Verification items for the finished model (mm, model axes). Face numbers are marked on the shaded views. A direction names the side the tool comes from. Round coordinates to 2 decimals unless told otherwise and drop trailing zeros. Order: outer loops, then holes, each group sorted by start corner. A loop starts at its lowest first (then second) coordinate and runs counter-clockwise, first axis right, second up. Notation, with made-up numbers: (-28.5, 69.5) -> (-9.5, 69.5) arc R19 cw to (-9.5, 74.5) -> close; hole circle Ø10 at (12.25, 71.5). An arc over 180 degrees is marked (long way). Return JSON: item names as keys, results as strings. Group by question number.
Item 1: Depth check by flat-ended pin: pin 1 Ø1.8 at (x, z) = (-5, -12.5) entering from -Y; pin 2 Ø3 at (x, y) = (6, 12) entering from -Z; pin 3 Ø12 at (x, y) = (2.5, 13.5) entering from +Z; pin 4 Ø2 at (y, z) = (9.5, -6.5) entering from -X. Enter the tip coordinate at first touch or a pass-through.
Item 2: Sectioned sample at A-A on z = 12.5. Record the cut outline in (x, y).
Item 3: Scan lines: probe 1 along Z at (x, y) = (-5.5, 3.5); probe 2 along X at (y, z) = (2.25, -12.5); probe 3 along Z at (x, y) = (-4.75, 14.25). Record each from-to range of solid material in increasing order. Write a range as from..to.
Item 4: Sectioned sample at C-C on y = 18. Record the cut outline in (x, z), plus the area to 3 significant figures.
Item 5: Access from +Z, -Z, +X, -X, +Y, -Y to the whole of each face (thin tool, end or side, straight path). Record for the marked faces 1, 2 and 3.
Item 6: Sectioned sample at B-B on x = -3. Record the cut outline in (y, z).
```python
from build123d import *

# Parameters (mm, degrees)
SKETCH_1_W          = 30
SKETCH_1_H          = 32
EXTRUDE_1_DEPTH     = 6
SKETCH_2_W          = 6
SKETCH_2_H          = 32
EXTRUDE_2_DEPTH     = 20
SKETCH_4_R          = 1.5
CUT_EXTRUDE_1_DEPTH = 30.681644159
SKETCH_5_W          = 24
SKETCH_5_H          = 5
EXTRUDE_3_DEPTH     = 20
CUT_EXTRUDE_2_DEPTH = 36.259750425


with BuildPart() as part:
    # 草图1 → 凸台-拉伸1 (new body)
    with BuildSketch(Plane(origin=(0, 0, 0), x_dir=(1, 0, 0), z_dir=(0, 1, 0))):
        Rectangle(SKETCH_1_W, SKETCH_1_H)
    extrude(amount=EXTRUDE_1_DEPTH)

    # 草图2 → 凸台-拉伸2 (add)
    with BuildSketch(Plane(origin=(0, 6, 0), x_dir=(1, 0, 0), z_dir=(0, 1, 0))):
        with Locations((12, 0)):
            Rectangle(SKETCH_2_W, SKETCH_2_H)
    extrude(amount=EXTRUDE_2_DEPTH)

    # 草图4 → 切除-拉伸1 (cut, through all)
    with BuildSketch(Plane(origin=(0, 6, 0), x_dir=(1, 0, 0), z_dir=(0, 1, 0))):
        with Locations(Location((-5, 12.5, 0), (0, 0, 270))):
            Circle(SKETCH_4_R)
        with Locations(Location((-5, -12.5, 0), (0, 0, 90))):
            Circle(SKETCH_4_R)
    extrude(amount=-CUT_EXTRUDE_1_DEPTH, mode=Mode.SUBTRACT)

    # 草图5 → 凸台-拉伸3 (add, through all)
    with BuildSketch(Plane(origin=(0, 6, 0), x_dir=(1, 0, 0), z_dir=(0, 1, 0))):
        with Locations((-3, 0)):
            Rectangle(SKETCH_5_W, SKETCH_5_H)
    extrude(amount=EXTRUDE_3_DEPTH)

    # 草图6 → 切除-拉伸2 (cut, through all)
    with BuildSketch(Plane.XY.offset(2.5)):
        Polygon((-15, 6), (-15, 26), (9, 26), align=None)
    extrude(amount=-CUT_EXTRUDE_2_DEPTH, mode=Mode.SUBTRACT)


solid = part.part
```
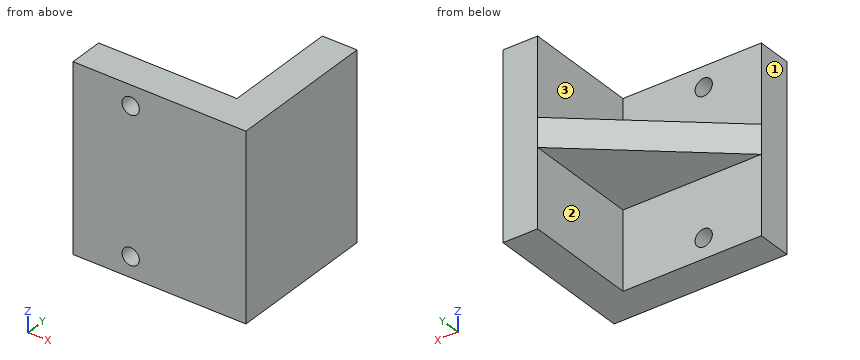
Recorded:
{
 "1": {"pin 1": "through", "pin 2": "z = -2.5", "pin 3": "z = 2.5", "pin 4": "x = 9"},
 "2": {"outline": "(-15, 0) -> (-6.5, 0) -> (-6.5, 6) -> (-15, 6) -> close; (-3.5, 0) -> (15, 0) -> (15, 26) -> (9, 26) -> (9, 6) -> (-3.5, 6) -> close"},
 "3": {"probe 1": "-16..-13.91, -11.09..11.09, 13.91..16", "probe 2": "-15..-6.5, -3.5..15", "probe 3": "-2.5..2.5"},
 "4": {"outline": "(-0.6, -2.5) -> (9, -2.5) -> (9, -16) -> (15, -16) -> (15, 16) -> (9, 16) -> (9, 2.5) -> (-0.6, 2.5) -> close", "area": "240 mm²"},
 "5": {"face 1": "+Z, -Z, -X, +Y, -Y", "face 2": "-Z, -X, +Y", "face 3": "+Z, -X, +Y"},
 "6": {"outline": "(0, -16) -> (6, -16) -> (6, -2.5) -> (16, -2.5) -> (16, 2.5) -> (6, 2.5) -> (6, 16) -> (0, 16) -> close"}
}
